from build123d import *

# Parameters (mm, degrees)
BOSS_EXTRUDE1_DEPTH      = 11.1125
DRAFT2_START             = 21.18139532
DRAFT2_OUTLINE_W         = 28
DRAFT2_OUTLINE_H         = 26
DRAFT2_DEPTH             = 1.91806369
BOSS_EXTRUDE2_DEPTH      = 3.175
BOSS_EXTRUDE2_DEPTH_BACK = 3.175
SKETCH7_R                = 9.525


# Read off the part's stored shape, not the designer's step: Draft2
with BuildPart() as part:
    # Sketch3 → Loft1 section 0
    with BuildSketch(Plane(origin=(0, 11.1125, 0), x_dir=(1, 0, 0), z_dir=(0, 1, 0))):
        with BuildLine():
            Line((6.01391392, -11.192562017), (12.7, -0.388078778))
            Line((12.7, -0.388078778), (6.68608608, 10.804483239))
            Line((6.68608608, 10.804483239), (-6.01391392, 11.192562017))
            Line((-6.01391392, 11.192562017), (-12.7, 0.388078778))
            Line((-12.7, 0.388078778), (-6.68608608, -10.804483239))
            Line((-6.68608608, -10.804483239), (6.01391392, -11.192562017))
        make_face()
    # Sketch2 for Loft1 → Loft1 section 1
    with BuildSketch(Plane(origin=(0, 0, 0), x_dir=(1, 0, 0), z_dir=(0, 1, 0))):
        with BuildLine():
            # circular arc as an exact rational Bezier (weights 1, cos(half-angle), 1)
            Bezier((6.011108127, -11.187340126), (12.47012196, -7.716825231), (12.694074813, -0.38789772), weights=[1, 0.866025404, 1])
            Bezier((12.694074813, -0.38789772), (12.918027667, 6.941029791), (6.682966686, 10.799442406), weights=[1, 0.866025404, 1])
            Bezier((6.682966686, 10.799442406), (0.447905706, 14.65785502), (-6.011108127, 11.187340126), weights=[1, 0.866025404, 1])
            Bezier((-6.011108127, 11.187340126), (-12.47012196, 7.716825231), (-12.694074813, 0.38789772), weights=[1, 0.866025404, 1])
            Bezier((-12.694074813, 0.38789772), (-12.918027667, -6.941029791), (-6.682966686, -10.799442406), weights=[1, 0.866025404, 1])
            Bezier((-6.682966686, -10.799442406), (-0.447905706, -14.65785502), (6.011108127, -11.187340126), weights=[1, 0.866025404, 1])
        make_face()
    loft()

    # Sketch3<2> → Boss-Extrude1 (add)
    with BuildSketch(Plane(origin=(0, 11.1125, 0), x_dir=(1, 0, 0), z_dir=(0, 1, 0))):
        Polygon((6.01391392, -11.192562017), (12.7, -0.388078778), (6.68608608, 10.804483239), (-6.01391392, 11.192562017), (-12.7, 0.388078778), (-6.68608608, -10.804483239), align=None)
    extrude(amount=BOSS_EXTRUDE1_DEPTH)

    # Draft2 outline → Draft2 (cut)
    with BuildSketch(Plane(origin=(0, 0, 0), x_dir=(0.999996456847854, -0.002651888614820864, 0.00023190194633995566), z_dir=(0.00266200896657633, 0.9961946980917459, -0.0871150802224119)).offset(DRAFT2_START)):
        with Locations((0, -2)):
            Rectangle(DRAFT2_OUTLINE_W, DRAFT2_OUTLINE_H)
    extrude(amount=DRAFT2_DEPTH, mode=Mode.SUBTRACT)

    # Sketch7 → Boss-Extrude2 (add, two sides: drawn at the far end of the back side and taken through both)
    with BuildSketch(Plane(origin=(0, 22.225, 0), x_dir=(1, 0, 0), z_dir=(0, 1, 0)).offset(-BOSS_EXTRUDE2_DEPTH_BACK)):
        with Locations(Location((0, 0, 0), (0, 0, 270))):
            Circle(SKETCH7_R)
    extrude(amount=BOSS_EXTRUDE2_DEPTH + BOSS_EXTRUDE2_DEPTH_BACK)


solid = part.part
CAD build for the part. Positions are in the model's coordinates, mm. A direction names the side the tool comes from. Give positions to 0.01 mm unless a question says otherwise; leave off trailing zeros. Write each loop counter-clockwise with the first axis right and the second up, starting at its lowest first coordinate (ties: lowest second). Pieces come first, ordered by that corner, then holes. Notation, with made-up numbers: (40.5, -39.75) - (62.5, -39.75) arc R37 ccw to (62.5, -2.75) - close; hole circle Ø6 at (-8, 65.5). An arc over 180 degrees is marked (long way). Put each result on its own line as item: value.
(1) Drop flat-ended pins along their axis: pin 1 Ø1.5 at (x, z) = (7, 2.5) entering from -Y; pin 2 Ø4 at (y, z) = (21, 7) entering from -X; pin 3 Ø3 at (x, y) = (9, 21) entering from -Z; pin 4 Ø10 at (x, y) = (8, 14) entering from +Z. Give the stop position or say it passes through.
Working result:
pin 1: y = 0
pin 2: x = -9.8
pin 3: z = -9.09
pin 4: z = 11.21
(2) Saw through at A-A (y = 13). List the corners of the cut face in (x, z), then the cut area to 3 significant figures.
Working result:
outline: (-12.7, -0.39) - (-6.01, -11.19) - (6.69, -10.8) - (12.7, 0.39) - (6.01, 11.19) - (-6.69, 10.8) - close
area: 419 mm^2
(3) Saw through at B-B (y = 22.75). List the corners of the cut face in (x, z) (3 decimals).
Working result:
outline: circle Ø19.05 at (0, 0)
(4) Tool access for faces 1 (the flat face through (-9.31, 16.12, -5.87)), 2 (the flat face through (-9.735, 16.591, 5.13)), 3 (the flat face through (9.735, 16.116, -5.13)), 4 (the flat face through (9.31, 16.59, 5.87)), 5 (the cylindrical face through (0.419, 23.4, -9.516)): list every direction of +Z, -Z, +X, -X, +Y, -Y with a clear straight run to the whole face (end or side of a thin tool).
Working result:
face 1: -Z, -X, +Y
face 2: +Z, -X, +Y
face 3: -Z, +X, +Y
face 4: +Z, +X, +Y
face 5: +Y
(5) Wall check: L1, parallel to Z at x = 6, y = 7; L2, parallel to Z at x = 7.25, y = 22.75; L3, parallel to Y at x = 7, z = 9.25. Give the ranges that are in metal, low to high.
Working result:
L1: -10.95 to 11.19
L2: -6.18 to 6.18
L3: 0 to 22.05
